Model file for the job. Use its own axes, mm. A direction names the side the tool comes from. Give positions to 0.01 mm unless a question says otherwise; leave off trailing zeros. Order: outer loops, then holes, each group sorted by start corner. A loop starts at its lowest first (then second) coordinate and runs counter-clockwise, first axis right, second up. Notation, with made-up numbers: M 3,81 L 48,81 A19 cw 48,86 Z; hole C -4,-30.75 d8. An arc over 180 degrees is marked long. Return JSON: item names as keys, results as strings. Group by question number.
1. Pin check, flat tips, straight feed: pin 1 (21 mm diameter, centred on x = -19, y = -23, fed in from +Z); pin 2 (1 mm diameter, centred on x = 21, y = -11, fed in from +Z); pin 3 (2.5 mm diameter, centred on y = -7.5, z = 5, fed in from +X); pin 4 (8 mm diameter, centred on x = -10, z = 14, fed in from -Y). Stop position of each tip, or through.
2. Slice it at D-D on z = 17. List the corners of the cut face in (x, y).
3. Slice it at A-A on y = -21.5. List the corners of the cut face in (x, z), then the cut area to 3 significant figures.
4. Slice it at B-B on x = 2. List the corners of the cut face in (y, z).
5. Slice it at C-C on y = -9. List the corners of the cut face in (x, z) (1 decimal).
6. Two-plate mould, pull along X, no slides. Class faces 5 (the face through (-16.323, -5, 17)), 6 (the face through (-9, -36.83, -25)), 7 (the face through (20.403, -18, 25)): released by +X, released by -X, zero draft, split by the parting line, or undercut.
7. 3-axis set-ups, long thin cutter, end or side, ignore diameter. For faces 1 (the face through (-11, -10.668, 12)), 2 (the face through (18.482, -18.157, 13.919)), 3 (the face through (-6.412, -5, 7)), 4 (the face through (-13, -10.668, 63)): which of +Z, -Z, +X, -X, +Y, -Y reach the whole face in a straight line?
8. Wall check: probe 1 along Z at (x, y) = (-23, -12); probe 2 along X at (y, z) = (-33, 21); probe 3 along X at (y, z) = (-27.5, 20). Give the ranges that are in metal, low to high. Write a range as [from, to].
from build123d import *

# Parameters (mm, degrees)
F1_DEPTH = 36.83
F2_W     = 9.9101620726
F2_H     = 20.4049523454
F2_R     = 11.0608053269
F2_R_2   = 8.4731634686
F3_DEPTH = 10.668


with BuildPart() as f1:
    # F0 (on Front) → F1 (new body)
    with BuildSketch(Plane.XZ):
        Polygon((34.9770523608, -44.1585220397), (-25.9413123131, 23.4637726098), (-25.9413123131, -44.1585220397), align=None)
    extrude(amount=F1_DEPTH)



with BuildPart() as f1b:
    # F0 (on Front) → F1, piece 2 (new body)
    with BuildSketch(Plane.XZ):
        Polygon((-25.9413123131, 54.0686920285), (-25.9413123131, 29.2932782322), (5.829508882, 0), (16.6140999645, 8.890000172), (20.4032789916, 19.0916396677), (20.4032789916, 31.6250808537), (13.699343428, 45.0329519808), (0, 54.0686920285), align=None)
    extrude(amount=F1_DEPTH)


with BuildPart() as f1_1:
    add(f1.part)

    add(f1b.part)  # F3 merges F1b
    # F2 (on Front) → F3 (join)
    with BuildSketch(Plane.XZ):
        with Locations((-11.3675410394, 12.7937035868)):
            Rectangle(F2_W, F2_H)
        with Locations((-13.1163941696, 53.8951084018)):
            Circle(F2_R)
        with Locations((-13.1163941696, 53.8951084018)):
            Circle(F2_R_2, mode=Mode.SUBTRACT)
    extrude(amount=F3_DEPTH)


solid = f1_1.part
Result:
{
 "1": {"pin 1": "stops at z = 54.07", "pin 2": "stops at z = -28.09", "pin 3": "stops at x = 13.41", "pin 4": "stops at y = -36.83"},
 "2": {"outline": "M -25.94,-36.83 L -20.12,-36.83 L -20.12,0 L -25.94,0 Z; M -16.32,-10.67 L -12.61,-10.67 L -12.61,-36.83 L 19.63,-36.83 L 19.63,0 L -16.32,0 Z"},
 "3": {"outline": "M -25.94,-44.16 L 34.98,-44.16 L -25.94,23.46 Z; M -25.94,29.29 L 5.83,0 L 16.61,8.89 L 20.4,19.09 L 20.4,31.63 L 13.7,45.03 L 0,54.07 L -25.94,54.07 Z", "area": "3,830 mm2"},
 "4": {"outline": "M -36.83,-44.16 L 0,-44.16 L 0,-7.55 L -36.83,-7.55 Z; M -36.83,3.53 L 0,3.53 L 0,52.75 L -36.83,52.75 Z"},
 "5": {"outline": "M -25.9,-44.2 L 35,-44.2 L -7.1,2.6 L -6.4,2.6 L -6.4,11.3 L 5.8,0 L 16.6,8.9 L 20.4,19.1 L 20.4,31.6 L 13.7,45 L 0,54.1 L -2.1,54.1 A11.1 ccw -24.2,54.1 L -25.9,54.1 L -25.9,29.3 L -16.3,20.4 L -16.3,12.8 L -25.9,23.5 Z; hole M -21.6,54.1 L -4.6,54.1 A8.5 ccw Z"},
 "6": {"face 5": "undercut", "face 6": "zero draft", "face 7": "released by +X"},
 "7": {"face 1": "-Y", "face 2": "+X, +Y, -Y", "face 3": "+Y, -Y", "face 4": "+Z, +X, -X, -Y"},
 "8": {"probe 1": "z = [-44.16, 20.2], [26.58, 54.07]", "probe 2": "x = [-25.94, -23.72], [-16.95, 20.4]", "probe 3": "x = [-25.94, -22.82], [-15.86, 20.4]"}
}
